The listing builds one solid part. Answer for the finished solid, in the listing's coordinates (mm). Face numbers are marked on the shaded views. A direction names the side the tool comes from. Give positions to 0.01 mm unless a question says otherwise; leave off trailing zeros. Order: outer loops, then holes, each group sorted by start corner. A loop starts at its lowest first (then second) coordinate and runs counter-clockwise, first axis right, second up. Notation, with made-up numbers: (62.5, -34) - (120.5, -34) arc R16 cw to (120.5, -24) - close; hole circle Ø8 at (31.25, 50.5). An arc over 180 degrees is marked (long way). Answer as a JSON object with one key per item and string values. Group by question number.
Q1. A cutting plane is placed at A-A, the plane y = 4. Give the vertices of the cut face in (x, z).
Q2. For the marked faces 1 and 2, determine the directions among +Z, -Z, +X, -X, +Y, -Y from which every point of the face is accessible in a straight line to the end or side of a thin tool.
Q3. A cutting plane is placed at B-B, the plane z = 21. Give the vertices of the cut face in (x, y), and give its area (3 significant figures).
Q4. Given pin 1 (0.9 mm diameter, centred on x = 6, y = 16, fed in from -Z); pin 2 (1 mm diameter, centred on x = 6, y = 10.5, fed in from -Z); pin 3 (1.5 mm diameter, centred on x = 2.5, y = 16, fed in from -Z); pin 4 (10 mm diameter, centred on y = 4.5, z = 20.5, fed in from -X), each flat-ended and moving along its own axis, determine where each tip first touches the part or whether it passes through.
Q5. Consider line 1 (Y direction, x = 5.75, z = 3.5); line 2 (Y direction, x = 2.75, z = 28); line 3 (Z direction, x = 5.25, y = 13.5). Determine where each line is inside the solid, lowest interval first.
Q6. A cutting plane is placed at C-C, the plane z = 57. Give the vertices of the cut face in (x, y), and give its area (3 significant figures).
from build123d import *

# Parameters (mm, degrees)
F0_R     = 1.55
F1_DEPTH = 7.7


with BuildPart() as f1:
    # F0 (on Right) → F1 (new body)
    with BuildSketch(Plane.YZ):
        with BuildLine():
            ThreePointArc((0.378257, 31.335913), (0.214732, 30.672765), (0.096856, 30))
            Line((0.096856, 30), (8, 30))
            Line((8, 30), (8, 33.225827))
            ThreePointArc((8, 33.225827), (8.87868, 35.347148), (11, 36.225827))
            Line((11, 36.225827), (10.841426, 36.225827))
            ThreePointArc((10.841426, 36.225827), (13.364842, 37.122221), (14.757271, 39.409641))
            ThreePointArc((14.757271, 39.409641), (14.799371, 39.495296), (14.877529, 39.550072))
            Line((14.877529, 39.550072), (16.67311, 40.225827))
            Line((16.67311, 40.225827), (14.841426, 41.123461))
            Line((14.841426, 41.123461), (14.841426, 42.400047))
            Line((14.841426, 42.400047), (14.841426, 43.676633))
            Line((14.841426, 43.676633), (14.841426, 44.917755))
            Line((14.841426, 44.917755), (14.841426, 46.194341))
            Line((14.841426, 46.194341), (14.841426, 47.293622))
            Line((14.841426, 47.293622), (14.841426, 48.534747))
            Line((14.841426, 48.534747), (14.841426, 49.740411))
            Line((14.841426, 49.740411), (14.841426, 51.016998))
            Line((14.841426, 51.016998), (14.841426, 52.293584))
            Line((14.841426, 52.293584), (14.841426, 53.676549))
            Line((14.841426, 53.676549), (14.841426, 54.953136))
            Line((14.841426, 54.953136), (14.841426, 56.265183))
            Line((14.841426, 56.265183), (14.841426, 57.754532))
            Line((14.841426, 57.754532), (14.841426, 59.24388))
            Line((14.841426, 59.24388), (16.67311, 59.24388))
            Line((16.67311, 59.24388), (15.413323, 60.263127))
            ThreePointArc((15.413323, 60.263127), (15.05882, 60.601418), (14.764118, 60.992907))
            ThreePointArc((14.764118, 60.992907), (14.582735, 61.163743), (14.341426, 61.225827))
            Line((14.341426, 61.225827), (9.597594, 61.225827))
            ThreePointArc((9.597594, 61.225827), (8.99445, 61.02346), (8.63542, 60.498262))
            Line((8.63542, 60.498262), (0.378257, 31.335913))
        make_face()
        with BuildLine():
            Line((0, 28.611568), (0, 1))
            ThreePointArc((0, 1), (0.292893, 0.292893), (1, 0))
            Line((1, 0), (2, 0))
            ThreePointArc((2, 0), (2.707107, 0.292893), (3, 1))
            Line((3, 1), (3, 15))
            ThreePointArc((3, 15), (3.87868, 17.12132), (6, 18))
            ThreePointArc((6, 18), (7.414214, 18.585786), (8, 20))
            Line((8, 20), (8, 30))
            Line((8, 30), (0.096856, 30))
            ThreePointArc((0.096856, 30), (0.024243, 29.307471), (0, 28.611568))
        make_face()
        with Locations((4, 21)):
            Circle(F0_R, mode=Mode.SUBTRACT)
        Polygon((14.841426, 42.400047), (14.841426, 41.123461), (16.67311, 41.123461), align=None)
        Polygon((14.841426, 43.676633), (14.841426, 42.400047), (16.67311, 42.400047), align=None)
        Polygon((14.841426, 44.917755), (14.841426, 43.676633), (16.67311, 43.676633), align=None)
        Polygon((14.841426, 46.194341), (14.841426, 44.917755), (16.67311, 44.917755), align=None)
        Polygon((14.841426, 47.293622), (14.841426, 46.194341), (16.67311, 46.194341), align=None)
        Polygon((16.67311, 49.740411), (14.841426, 51.016998), (14.841426, 49.740411), align=None)
        Polygon((14.841426, 48.534747), (14.841426, 47.293622), (16.67311, 47.293622), align=None)
        Polygon((14.841426, 49.740411), (14.841426, 48.534747), (16.67311, 48.534747), align=None)
        Polygon((16.67311, 51.016998), (14.841426, 52.293584), (14.841426, 51.016998), align=None)
        Polygon((16.67311, 52.293584), (14.841426, 53.676549), (14.841426, 52.293584), align=None)
        Polygon((16.67311, 53.676549), (14.841426, 54.953136), (14.841426, 53.676549), align=None)
        Polygon((16.67311, 54.953136), (14.841426, 56.265183), (14.841426, 54.953136), align=None)
        Polygon((16.67311, 56.265183), (14.841426, 57.754532), (14.841426, 56.265183), align=None)
        Polygon((16.67311, 57.754532), (14.841426, 59.24388), (14.841426, 57.754532), align=None)
    extrude(amount=F1_DEPTH)


solid = f1.part
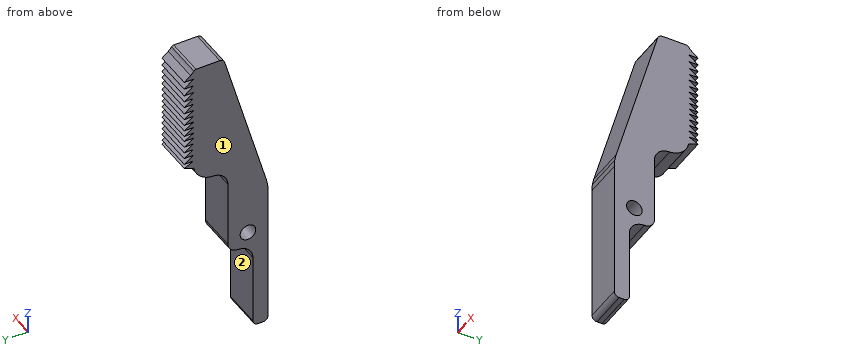
Reply:
{
 "1": {"outline": "(0, 17.24) - (7.7, 17.24) - (7.7, 19.45) - (0, 19.45) - close; (0, 22.55) - (7.7, 22.55) - (7.7, 44.13) - (0, 44.13) - close"},
 "2": {"face 1": "+Z, -Z, -X, +Y, -Y", "face 2": "-Z, +X, -X, +Y"},
 "3": {"outline": "(0, 0) - (7.7, 0) - (7.7, 2.45) - (0, 2.45) - close; (0, 5.55) - (7.7, 5.55) - (7.7, 8) - (0, 8) - close", "area": "37.7 mm^2"},
 "4": {"pin 1": "stops at z = 39.8", "pin 2": "stops at z = 36.05", "pin 3": "stops at z = 39.69", "pin 4": "stops at x = 0"},
 "5": {"line 1": "y = 0 to 3", "line 2": "y = 0 to 8", "line 3": "z = 37.24 to 61.23"},
 "6": {"outline": "(0, 7.64) - (7.7, 7.64) - (7.7, 15.77) - (0, 15.77) - close", "area": "62.6 mm^2"}
}
